Build history of the part. All positions in model axes, mm. Coordinates: 2 decimals unless noted, no trailing zeros. Write each loop counter-clockwise with the first axis right and the second up, starting at its lowest first coordinate (ties: lowest second). Pieces come first, ordered by that corner, then holes. Notation, with made-up numbers: (75.5, 58.5) -> (115.5, 58.5) arc R31 cw to (115.5, 87.5) -> close; hole circle Ø2 at (54, 3). An arc over 180 degrees is marked (long way). Write each question's results on one line, items separated by ' | '. Start each with the question number.
Q1. Drill centre lines: line 1 (Y direction, x = -2.5, z = 209.5); line 2 (X direction, y = -4, z = 407). Where is each one in solid material? Low to high.
Q2. Saw through at A-A on x = -22.5. Count the separate pieces of the cut face and the enclosed holes in it, and give its area (3 significant figures).
Q3. Saw through at C-C on z = 193. Give the cut face in (x, y), and give its area (3 significant figures).
Q4. Saw through at B-B on z = 273.5. Give the cut face in (x, y).
Q5. Drop flat-ended pins along their axis: pin 1 Ø7.5 at (x, z) = (-16, 111.5) entering from -Y; pin 2 Ø3.5 at (x, y) = (-22, -16) entering from +Z; pin 3 Ø3.5 at (x, y) = (-20.5, -15.5) entering from -Z. Give the stop position or say it passes through.
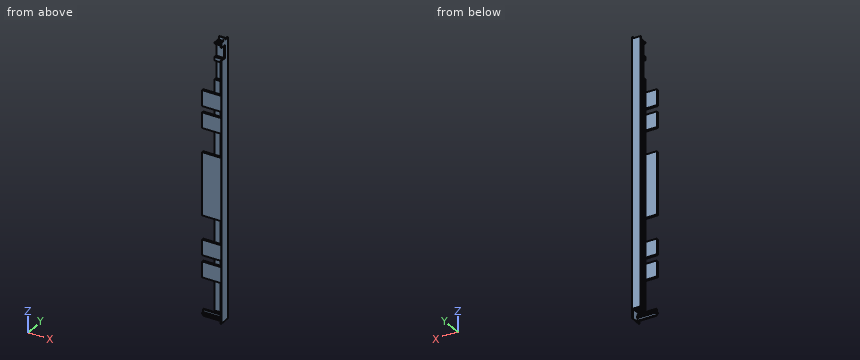
from build123d import *

# Parameters (mm, degrees)
EXTRUDE_1_DEPTH          = 449.532
SKETCH_7_W               = 15
SKETCH_7_H               = 12.9
CUT_EXTRUDE_2_DEPTH      = 12.5
CUT_EXTRUDE_3_DEPTH      = 12.5
SKETCH_10_W              = 25.5
SKETCH_10_H              = 3
SKETCH_10_W_2            = 101
SKETCH_10_W_3            = 25
EXTRUDE_6_DEPTH          = 30
CUT_EXTRUDE_4_DEPTH      = 30
CUT_EXTRUDE_4_DEPTH_BACK = 30
SKETCH_11_W              = 21
SKETCH_11_H              = 9
SKETCH_12_W              = 30
SKETCH_12_H              = 4
CUT_EXTRUDE_5_DEPTH      = 12.5
SKETCH_15_W              = 7
SKETCH_15_H              = 2
CUT_EXTRUDE_8_DEPTH      = 12.5
SKETCH_17_W              = 20
SKETCH_17_H              = 2.5
CUT_EXTRUDE_9_DEPTH      = 12.5
FILLET_2_R               = 1
FILLET_3_R               = 1
FILLET_4_R               = 1


with BuildPart() as part:
    # 草图1 → 凸台-拉伸1 (new body)
    with BuildSketch(Plane.XY):
        Polygon((0, 0), (-14, 0), (-14, -1), (-1.5, -1), (-1.5, -3.55), (-14, -3.55), (-14, -7.25), (-1.5, -7.25), (-1.5, -8.9), (-14, -8.9), (-14, -12.9), (-1.5, -12.9), (-1.5, -17.9), (0, -17.9), align=None)
    extrude(amount=EXTRUDE_1_DEPTH)

    # 草图7 → 切除-拉伸2 (cut)
    with BuildSketch(Plane.ZY.offset(14)):
        with Locations((7.5, -6.45)):
            Rectangle(SKETCH_7_W, SKETCH_7_H)
    extrude(amount=-CUT_EXTRUDE_2_DEPTH, mode=Mode.SUBTRACT)

    # 草图8 → 切除-拉伸3 (cut)
    with BuildSketch(Plane.ZY.offset(14)):
        Polygon((449.532, -12.9), (443.032, -12.9), (443.032, -1), (446.532, -1.000447275), (446.532, 0), (449.532, 0), align=None)
    extrude(amount=-CUT_EXTRUDE_3_DEPTH, mode=Mode.SUBTRACT)

    # 草图10 → 凸台-拉伸6 (add)
    with BuildSketch(Plane.ZY.offset(1.5)):
        Polygon((6.5, -14.9), (6.5, -16.9), (8.5, -16.9), (8.5, -14.9), (12.5, -14.9), (12.5, -12.9), (8.5, -12.9), (8.5, -10.9), (6.5, -10.9), (6.5, -12.9), (2.5, -12.9), (2.5, -14.9), align=None)
        with Locations((77.25, -15.4)):
            Rectangle(SKETCH_10_W, SKETCH_10_H)
        with Locations((214.017, -15.4)):
            Rectangle(SKETCH_10_W_2, SKETCH_10_H)
        with Locations((112.5, -15.4)):
            Rectangle(SKETCH_10_W_3, SKETCH_10_H)
        with Locations((315.532, -15.4)):
            Rectangle(SKETCH_10_W_3, SKETCH_10_H)
        with Locations((350.782, -15.4)):
            Rectangle(SKETCH_10_W, SKETCH_10_H)
    extrude(amount=EXTRUDE_6_DEPTH)

    # 草图11 → 切除-拉伸4 (cut, two sides: drawn at the far end of the back side and taken through both)
    with BuildSketch(Plane.ZY.offset(1.5).offset(-CUT_EXTRUDE_4_DEPTH_BACK)):
        with Locations((430.4789, -13.4)):
            Rectangle(SKETCH_11_W, SKETCH_11_H)
    extrude(amount=CUT_EXTRUDE_4_DEPTH + CUT_EXTRUDE_4_DEPTH_BACK, mode=Mode.SUBTRACT)

    # 草图12 → 切除-拉伸5 (cut)
    with BuildSketch(Plane.ZY.offset(14)):
        with Locations((399.0289, -10.9)):
            Rectangle(SKETCH_12_W, SKETCH_12_H)
    extrude(amount=-CUT_EXTRUDE_5_DEPTH, mode=Mode.SUBTRACT)

    # 草图15 → 切除-拉伸8 (cut)
    with BuildSketch(Plane.ZY.offset(14)):
        with Locations((34.5, -9.9)):
            Rectangle(SKETCH_15_W, SKETCH_15_H)
    extrude(amount=-CUT_EXTRUDE_8_DEPTH, mode=Mode.SUBTRACT)

    # 草图17 → 切除-拉伸9 (cut)
    with BuildSketch(Plane.ZY.offset(14)):
        with Locations((67, -10.15)):
            Rectangle(SKETCH_17_W, SKETCH_17_H)
    extrude(amount=-CUT_EXTRUDE_9_DEPTH, mode=Mode.SUBTRACT)

    # 圆角2
    fillet_2_edges = [part.edges().sort_by_distance(p)[0] for p in [
        (0, 0, 224.766),
    ]]
    fillet(fillet_2_edges, radius=FILLET_2_R)

    # 圆角3
    fillet_3_edges = [part.edges().sort_by_distance(p)[0] for p in [
        (0, -9.45, 0),
        (-1.25, 0, 0),
        (-0.292893219, -0.292893219, 0),
    ]]
    fillet(fillet_3_edges, radius=FILLET_3_R)

    # 圆角4
    fillet_4_edges = [part.edges().sort_by_distance(p)[0] for p in [
        (-1.25, 0, 449.532),
        (-0.292893219, -0.292893219, 449.532),
        (0, -9.45, 449.532),
    ]]
    fillet(fillet_4_edges, radius=FILLET_4_R)


solid = part.part
Returned:
1) line 1: y = -16.9 to -13.9, -12.9 to -8.9, -7.25 to -3.55, -1 to 0 | line 2: x = -14 to 0
2) separate pieces: 6 | enclosed holes: 0 | area: 634 mm2
3) outline: (-31.5, -16.9) -> (-1.5, -16.9) -> (-1.5, -17.9) -> (0, -17.9) -> (0, -1) arc R1 ccw to (-1, 0) -> (-14, 0) -> (-14, -1) -> (-1.5, -1) -> (-1.5, -3.55) -> (-14, -3.55) -> (-14, -7.25) -> (-1.5, -7.25) -> (-1.5, -8.9) -> (-14, -8.9) -> (-14, -12.9) -> (-1.5, -12.9) -> (-1.5, -13.9) -> (-31.5, -13.9) -> close | area: 225 mm2
4) outline: (-14, -12.9) -> (-1.5, -12.9) -> (-1.5, -17.9) -> (0, -17.9) -> (0, -1) arc R1 ccw to (-1, 0) -> (-14, 0) -> (-14, -1) -> (-1.5, -1) -> (-1.5, -3.55) -> (-14, -3.55) -> (-14, -7.25) -> (-1.5, -7.25) -> (-1.5, -8.9) -> (-14, -8.9) -> close
5) pin 1: stops at y = -16.9 | pin 2: stops at z = 363.53 | pin 3: stops at z = 2.5
